Check sheet for the modelled part. Datum: model origin and axes. Units: mm. Face numbers are marked on the shaded views. A direction names the side the tool comes from. Give positions to 0.01 mm unless a question says otherwise; leave off trailing zeros. Loops run counter-clockwise (first coordinate to the right, second up) from the corner with the lowest first, then second, coordinate; pieces in that order, holes last. Notation, with made-up numbers: M 7,-31 L 60,-31 A15 ccw 60,-23 Z; hole C 34,83.25 d7. An arc over 180 degrees is marked long. Put each result on its own line as item: value. Start each with the question number.
```python
from build123d import *

# Parameters (mm, degrees)
SKETCH1_R                   = 12
BOSS_EXTRUDE1_DEPTH         = 33
FILLET1_R                   = 10
M8_TAPPED_HOLE2_D           = 8
M8_TAPPED_HOLE2_DEPTH       = 33
M8_TAPPED_HOLE2_CSINK_D     = 8.05
M8_TAPPED_HOLE2_CSINK_ANGLE = 90
CUT_EXTRUDE1_REACH          = 35


with BuildPart() as part:
    # Sketch1 → Boss-Extrude1 (new body)
    with BuildSketch(Plane(origin=(0, 0, 0), x_dir=(1, 0, 0), z_dir=(0, 1, 0))):
        with BuildLine():
            Line((125, 0), (-125, 0))
            Line((-125, 0), (-125, 123.505102572))
            ThreePointArc((-125, 123.505102572), (-120.023162168, 176.706671295), (-68.377223398, 163))
            Line((-68.377223398, 163), (68.377223398, 163))
            ThreePointArc((68.377223398, 163), (120.023162168, 176.706671295), (125, 123.505102572))
            Line((125, 123.505102572), (125, 0))
        make_face()
        with Locations((-100, 148)):
            Circle(SKETCH1_R, mode=Mode.SUBTRACT)
        with Locations((100, 148)):
            Circle(SKETCH1_R, mode=Mode.SUBTRACT)
    extrude(amount=BOSS_EXTRUDE1_DEPTH)

    # Fillet1
    fillet1_edges = [part.edges().sort_by_distance(p)[0] for p in [
        (-125, 16.5, -123.505102572),
        (-68.377223398, 16.5, -163),
        (68.377223398, 16.5, -163),
        (125, 16.5, -123.505102572),
    ]]
    fillet(fillet1_edges, radius=FILLET1_R)

    # M8 Tapped Hole2
    with Locations(Plane(origin=(0, 33, 0), x_dir=(1, 0, 0), z_dir=(0, 1, 0))):
        with Locations((-53, 85), (53, 85), (53, 14), (-53, 14)):
            CounterSinkHole(M8_TAPPED_HOLE2_D / 2, M8_TAPPED_HOLE2_CSINK_D / 2, depth=M8_TAPPED_HOLE2_DEPTH, counter_sink_angle=M8_TAPPED_HOLE2_CSINK_ANGLE)

    # Sketch6 → Cut-Extrude1 (cut, up to next)
    with BuildSketch(Plane(origin=(0, 33, 0), x_dir=(1, 0, 0), z_dir=(0, 1, 0)), mode=Mode.PRIVATE) as cut_extrude1_sk1:
        with BuildLine():
            Line((-43.216947182, 65.77208412), (36.783052818, 65.77208412))
            ThreePointArc((36.783052818, 65.77208412), (51.783052818, 50.77208412), (36.783052818, 35.77208412))
            Line((36.783052818, 35.77208412), (-43.216947182, 35.77208412))
            ThreePointArc((-43.216947182, 35.77208412), (-58.216947182, 50.77208412), (-43.216947182, 65.77208412))
        make_face()
    cut_extrude1_tool1 = extrude(cut_extrude1_sk1.sketch, amount=-CUT_EXTRUDE1_REACH, mode=Mode.PRIVATE) & part.part
    add(cut_extrude1_tool1.solids().sort_by_distance((-3.216947, 33, -50.772084))[0], mode=Mode.SUBTRACT)


solid = part.part
```
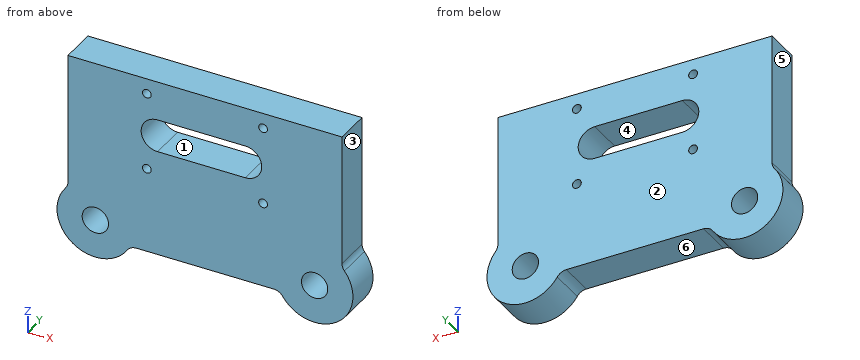
Q1. Access from +Z, -Z, +X, -X, +Y, -Y to the whole of each face (thin tool, end or side, straight path). Record for the marked faces 1, 2 and 3.
Q2. Thickness scan on line 1 along Z through (x, y) = (53, 18); line 2 along X through (y, z) = (9, -85); line 3 along X through (y, z) = (13, -148). Record the ranges inside material, lowest first. Write a range as [from, to].
Q3. Section check B-B, the plane z = -148. Record the cut outline in (x, y), then the cut area to 3 significant figures.
Q4. Mould release check, pull along Z, two halves, no side actions. Record for the marked faces 4, 5 and 6: pulls with the +Z half, pulls with the -Z half, needs draft (parallel to the pull), parting line crosses it, or undercut.
Q5. Depth check by flat-ended pin: P1, Ø1.5, axis at x = 36, z = -137.5, coming from the -Y side; P2, Ø6.5, axis at x = 53, z = -14, coming from the -Y side; P3, Ø8, axis at x = -91, y = 27.5, coming from the -Z side; P4, Ø10, axis at y = 12, z = -40.5, coming from the +X side. Enter the tip coordinate at first touch or a pass-through.
Q6. Section check C-C, the plane y = 19. Record the cut outline in (x, z), then the cut area to 3 significant figures.
Q7. Section check D-D, the plane x = -53. Record the cut outline in (y, z) (3 decimals).
Q8. Section check A-A, the plane x = 100. Record the cut outline in (y, z), then the cut area to 3 significant figures.
Found:
1. face 1: +Y, -Y
1. face 2: +Z, -Z, +X, -X, +Y
1. face 3: +Z, +X, +Y, -Y
2. line 1: z = [-163, -89], [-81, -18], [-10, 0]
2. line 2: x = [-125, -57], [-49, 49], [57, 125]
2. line 3: x = [-135, -112], [-88, 88], [112, 135]
3. outline: M -135,0 L -112,0 L -112,33 L -135,33 Z; M -88,0 L 88,0 L 88,33 L -88,33 Z; M 112,0 L 135,0 L 135,33 L 112,33 Z
3. area: 7,330 mm^2
4. face 4: undercut
4. face 5: needs draft
4. face 6: pulls with the -Z half
5. P1: stops at y = 0
5. P2: passes through
5. P3: stops at z = -182.64
5. P4: stops at x = 125
6. outline: M -127.22,-126 A35 ccw long -70.9,-167.44 A10 cw -62.58,-163 L 62.58,-163 A10 cw 70.9,-167.44 A35 ccw long 127.22,-126 A10 cw 125,-119.72 L 125,0 L -125,0 L -125,-119.72 A10 cw Z; hole C -100,-148 d24; hole C -53,-85 d8; hole C -53,-14 d8; hole M -43.22,-65.77 L 36.78,-65.77 A15 ccw 36.78,-35.77 L -43.22,-35.77 A15 ccw Z; hole C 53,-85 d8; hole C 53,-14 d8; hole C 100,-148 d24
6. area: 39,000 mm^2
7. outline: M 0,-163 L 33,-163 L 33,-89.025 L 32.975,-89 L 0,-89 Z; M 0,-81 L 32.975,-81 L 33,-80.975 L 33,-62.143 L 0,-62.143 Z; M 0,-39.401 L 33,-39.401 L 33,-18.025 L 32.975,-18 L 0,-18 Z; M 0,-10 L 32.975,-10 L 33,-9.975 L 33,0 L 0,0 Z
8. outline: M 0,-183 L 33,-183 L 33,-160 L 0,-160 Z; M 0,-136 L 33,-136 L 33,0 L 0,0 Z
8. area: 5,250 mm^2
